Geometry check sheet. Reference: the model listing, model coordinates, mm. A direction names the side the tool comes from. Give positions to 0.01 mm unless a question says otherwise; leave off trailing zeros. Order: outer loops, then holes, each group sorted by start corner. A loop starts at its lowest first (then second) coordinate and runs counter-clockwise, first axis right, second up.
from build123d import *

# Parameters (mm, degrees)
SKETCH1_W           = 12
SKETCH1_H           = 6
BOSS_EXTRUDE1_DEPTH = 6


with BuildPart() as part:
    # Sketch1 → Boss-Extrude1 (new body)
    with BuildSketch(Plane(origin=(0, 0, 0), x_dir=(0, 0, -1), z_dir=(1, 0, 0))):
        with BuildLine():
            Line((86.321496787, 73.422774132), (60.826091075, 73.422774132))
            Line((60.826091075, 73.422774132), (60.060334343, 69.316135154))
            ThreePointArc((60.060334343, 69.316135154), (51.261909479, 37.228978051), (37.265778766, 7.044441347))
            Line((37.265778766, 7.044441347), (18.112573434, -26.605921739))
            Line((18.112573434, -26.605921739), (10.903253971, -26.605921739))
            Line((10.903253971, -26.605921739), (10.903253971, -45.622400338))
            Line((10.903253971, -45.622400338), (15.367545377, -45.622400338))
            Line((15.367545377, -45.622400338), (15.367545377, -53.626330222))
            Line((15.367545377, -53.626330222), (24.367545377, -53.626330222))
            Line((24.367545377, -53.626330222), (24.367545377, -45.622400338))
            Line((24.367545377, -45.622400338), (33.453304177, -45.622400338))
            Line((33.453304177, -45.622400338), (33.453304177, -37.622400338))
            Line((33.453304177, -37.622400338), (39.453304177, -37.622400338))
            Line((39.453304177, -37.622400338), (39.453304177, -45.622400338))
            Line((39.453304177, -45.622400338), (58.367545377, -45.622400338))
            Line((58.367545377, -45.622400338), (58.367545377, -72.9735186))
            Line((58.367545377, -72.9735186), (73.367545377, -72.9735186))
            Line((73.367545377, -72.9735186), (73.367545377, -45.622400338))
            Line((73.367545377, -45.622400338), (86.321496787, -45.622400338))
            Line((86.321496787, -45.622400338), (86.321496787, -35.622400338))
            Line((86.321496787, -35.622400338), (80.321496787, -35.622400338))
            Line((80.321496787, -35.622400338), (80.321496787, -23.622400338))
            Line((80.321496787, -23.622400338), (86.321496787, -23.622400338))
            Line((86.321496787, -23.622400338), (86.321496787, -5.622400338))
            Line((86.321496787, -5.622400338), (80.321496787, -5.622400338))
            Line((80.321496787, -5.622400338), (80.321496787, 2.377599662))
            Line((80.321496787, 2.377599662), (86.321496787, 2.377599662))
            Line((86.321496787, 2.377599662), (86.321496787, 73.422774132))
        make_face()
        with Locations((70.374836387, 65.422774132)):
            Rectangle(SKETCH1_W, SKETCH1_H, mode=Mode.SUBTRACT)
        with Locations((70.374836387, 53.422774132)):
            Rectangle(SKETCH1_W, SKETCH1_H, mode=Mode.SUBTRACT)
    extrude(amount=BOSS_EXTRUDE1_DEPTH)


solid = part.part
Item 1: Gauge pin test, flat ends, axial feed: pin 1 (1.8 mm diameter, centred on x = 4, z = -21, fed in from -Y); pin 2 (1.8 mm diameter, centred on x = 3.5, z = -53, fed in from -Y); pin 3 (1.8 mm diameter, centred on x = 3.5, y = -60.5, fed in from -Z). Record the tip position at first contact, or that the pin passes through.
Reported:
pin 1: stops at y = -53.63
pin 2: stops at y = -45.62
pin 3: stops at z = -73.37
Item 2: Set-up check for faces 1 (the flat face through (3, -45.622, -80)), 2 (the flat face through (3, 68.423, -70)), 3 (the flat face through (3, -42, -33.453)), 4 (the flat face through (3, 37, -86.321)), 5 (the flat face through (3, -2, -80.321)): record each of +Z, -Z, +X, -X, +Y, -Y from which the full face is reachable in a straight line by a thin tool's end or side.
Reported:
face 1: -Z, +X, -X, -Y
face 2: +X, -X
face 3: +X, -X, -Y
face 4: -Z, +X, -X, +Y, -Y
face 5: -Z, +X, -X
Item 3: Sectioned sample at B-B (x = 4.2). Give the number of separate pieces and of enclosed holes in the cut face, and give its area (3 significant figures).
Reported:
separate pieces: 1
enclosed holes: 2
area: 5,910 mm2
Item 4: Draft check along Z on faces 6 (the flat face through (3, -50, -15.368)), 7 (the flat face through (3, -35.622, -83)), 8 (the flat face through (3, 62.423, -70)), 9 (the flat face through (3, -30, -80.321)). Enter one of: released by +Z, released by -Z, zero draft, split by the parting line, or undercut.
Reported:
face 6: released by +Z
face 7: zero draft
face 8: undercut
face 9: released by -Z
Item 5: Scan lines: L1, parallel to Y at x = 4.8, z = -66.5; L2, parallel to Y at x = 2.05, z = -73.5; L3, parallel to Y at x = 4.1, z = -15. Record each from-to range of solid material in increasing order.
Reported:
L1: y = -72.97 to 50.42, 56.42 to 62.42, 68.42 to 73.42
L2: y = -45.62 to 50.42, 56.42 to 62.42, 68.42 to 73.42
L3: y = -45.62 to -26.61
Item 6: Sectioned sample at A-A (y = -43.5). Enter the section's corners in (x, z).
Reported:
outline: (0, -86.32) - (6, -86.32) - (6, -39.45) - (0, -39.45) - close; (0, -33.45) - (6, -33.45) - (6, -10.9) - (0, -10.9) - close
Item 7: Sectioned sample at C-C (y = -59). Enter the section's corners in (x, z), and give its area (3 significant figures).
Reported:
outline: (0, -73.37) - (6, -73.37) - (6, -58.37) - (0, -58.37) - close
area: 90.0 mm2
Item 8: Sectioned sample at D-D (z = -30). Enter the section's corners in (x, y).
Reported:
outline: (0, -45.62) - (6, -45.62) - (6, -5.72) - (0, -5.72) - close
